CAD build for the part. Positions are in the model's coordinates, mm. A direction names the side the tool comes from. Give positions to 0.01 mm unless a question says otherwise; leave off trailing zeros. Loops run counter-clockwise (first coordinate to the right, second up) from the corner with the lowest first, then second, coordinate; pieces in that order, holes last.
Item 1: Drop flat-ended pins along their axis: P1, Ø1.5, axis at x = -38.5, z = 38.5, coming from the -Y side; P2, Ø4, axis at x = 9.5, y = -11.5, coming from the +Z side; P3, Ø7, axis at x = -38, y = 5.5, coming from the +Z side. Give the stop position or say it passes through.
Item 2: Saw through at A-A on y = -8. Give the cut face in (x, z).
Item 3: Saw through at B-B on x = -40.5. Give the cut face in (y, z).
Item 4: Saw through at D-D on y = 4.5. Give the cut face in (x, z).
Item 5: Mould opens along X. For faces 4 (the flat face through (50, 0, 5)), 5 (the flat face through (0, 5, 45)), 6 (the flat face through (15, 3, 40)), 7 (the flat face through (-46.012, 4, 37)) say: released by +X, released by -X, zero draft, split by the parting line, or undercut.
Item 6: Which spindle directions (+Z, -Z, +X, -X, +Y, -Y) get a long thin tool onto all of the face, cutting with end or side? Do faces 1 (the flat face through (-15, 3, 40)), 2 (the flat face through (-41, 0, 37)), 3 (the flat face through (-41, 4, 40)). Say none if no direction does.
Item 7: Probe probe 1 along Z at (x, y) = (16, 11.5); probe 2 along Y at (x, z) = (36, 29); probe 3 along Z at (x, y) = (35, -2.5). List the from-to ranges inside material, lowest first.
Item 8: Saw through at C-C on z = 0. Give the cut face in (x, y), plus the area to 3 significant figures.
from build123d import *

# Parameters (mm, degrees)
F0_W      = 100
F0_H      = 50
F1_DEPTH  = 15
F3_R      = 25
F4_DEPTH  = 20
F2_W      = 30
F2_H      = 10
F5_DEPTH  = 100
F6_R      = 10
F7_DEPTH  = 5
F8_W      = 11.012334
F8_H      = 8.445302
F9_DEPTH  = 5
F10_W     = 30
F10_H     = 30
F11_DEPTH = 10
F13_DEPTH = 65.001


with BuildPart() as f1:
    # F0 (on Front) → F1 (new body, symmetric)
    with BuildSketch(Plane.XZ):
        Rectangle(F0_W, F0_H)
    extrude(amount=F1_DEPTH, both=True)

    # F3 (on face) → F4 (join)
    with BuildSketch(Plane.XZ.offset(15)):
        Circle(F3_R)
    extrude(amount=F4_DEPTH)

    # F2 (on face) → F5 (join)
    with BuildSketch(Plane.YZ.offset(50)):
        with Locations((0, 30)):
            Rectangle(F2_W, F2_H)
    extrude(amount=-F5_DEPTH)

    # F6 (on face) → F7 (join)
    with BuildSketch(Plane.XY.offset(35)):
        with Locations((35, 0)):
            Circle(F6_R)
    extrude(amount=F7_DEPTH)

    # F8 (on face) → F9 (join)
    with BuildSketch(Plane.XY.offset(35)):
        with Locations((-40.506167, 4.222651)):
            Rectangle(F8_W, F8_H)
    extrude(amount=F9_DEPTH)

    # F10 (on face) → F11 (join)
    with BuildSketch(Plane.XY.offset(35)):
        Rectangle(F10_W, F10_H)
    extrude(amount=F11_DEPTH)

    # F12 (on face) → F13 (cut, through all)
    with BuildSketch(Plane.YZ.offset(15)):
        Polygon((-15, 45), (-15, 35), (-5, 45), align=None)
    extrude(amount=-F13_DEPTH, mode=Mode.SUBTRACT)


solid = f1.part
Results below:
1. P1: stops at y = 0
1. P2: stops at z = 40.5
1. P3: stops at z = 40
2. outline: (-50, -25) - (50, -25) - (50, 35) - (41, 35) - (41, 40) - (29, 40) - (29, 35) - (15, 35) - (15, 42) - (-15, 42) - (-15, 35) - (-50, 35) - close
3. outline: (-15, -25) - (15, -25) - (15, 35) - (8.45, 35) - (8.45, 40) - (0, 40) - (0, 35) - (-15, 35) - close
4. outline: (-50, -25) - (50, -25) - (50, 35) - (43.93, 35) - (43.93, 40) - (26.07, 40) - (26.07, 35) - (15, 35) - (15, 45) - (-15, 45) - (-15, 35) - (-35, 35) - (-35, 40) - (-46.01, 40) - (-46.01, 35) - (-50, 35) - close
5. face 4: released by +X
5. face 5: zero draft
5. face 6: undercut
5. face 7: released by -X
6. face 1: +Z, +Y, -Y
6. face 2: +Z, -X, -Y
6. face 3: +Z, -X, +Y, -Y
7. probe 1: z = -25 to 35
7. probe 2: y = -15 to 15
7. probe 3: z = -25 to 40
8. outline: (-50, -15) - (-25, -15) - (-25, -35) - (25, -35) - (25, -15) - (50, -15) - (50, 15) - (-50, 15) - close
8. area: 4,000 mm2
